```python
from build123d import *

# Parameters (mm, degrees)
SKETCH1_W           = 7.5
SKETCH1_H           = 7.5
BOSS_EXTRUDE1_DEPTH = 7.5
SKETCH2_W           = 5.5
SKETCH2_H           = 6.5
CUT_EXTRUDE1_DEPTH  = 6.5
CUT_EXTRUDE2_REACH  = 13.25
SKETCH4_R           = 1.3
CUT_EXTRUDE3_DEPTH  = 1
SKETCH5_R           = 1.5
CUT_EXTRUDE4_DEPTH  = 0.2
FILLET1_R           = 1


with BuildPart() as part:
    # Sketch1 → Boss-Extrude1 (new body)
    with BuildSketch(Plane(origin=(0, 0, 0), x_dir=(1, 0, 0), z_dir=(0, 1, 0))):
        Rectangle(SKETCH1_W, SKETCH1_H)
    extrude(amount=BOSS_EXTRUDE1_DEPTH)

    # Sketch2 → Cut-Extrude1 (cut)
    with BuildSketch(Plane(origin=(0, 7.5, 0), x_dir=(1, 0, 0), z_dir=(0, 1, 0))):
        with Locations((0, -0.5)):
            Rectangle(SKETCH2_W, SKETCH2_H)
    extrude(amount=-CUT_EXTRUDE1_DEPTH, mode=Mode.SUBTRACT)

    # Cut-Extrude2: up to this face of the body (flat: up to its plane)
    cut_extrude2_end = Plane(part.part.faces().sort_by_distance((-3.75, 3.75, 0))[0])
    # Sketch3 → Cut-Extrude2 (cut, up to the picked face)
    with BuildSketch(Plane(origin=(3.75, 0, 0), x_dir=(0, 0, -1), z_dir=(1, 0, 0)), mode=Mode.PRIVATE) as cut_extrude2_sk1:
        Polygon((-3.75, 7.5), (2.75, 7.5), (-3.75, 1), align=None)
    cut_extrude2_tool1 = split(extrude(cut_extrude2_sk1.sketch, amount=-CUT_EXTRUDE2_REACH, mode=Mode.PRIVATE), bisect_by=cut_extrude2_end, keep=Keep.BOTH, mode=Mode.PRIVATE)
    add(cut_extrude2_tool1.solids().sort_by(Axis((3.75, 5.333333, 1.583333), (-1, 0, 0)))[0], mode=Mode.SUBTRACT)

    # Sketch4 → Cut-Extrude3 (cut)
    with BuildSketch(Plane.XZ):
        with Locations(Location((0, 0, 0), (0, 0, 270))):
            Circle(SKETCH4_R)
    extrude(amount=-CUT_EXTRUDE3_DEPTH, mode=Mode.SUBTRACT)

    # Sketch5 → Cut-Extrude4 (cut)
    with BuildSketch(Plane(origin=(0, 1, 0), x_dir=(1, 0, 0), z_dir=(0, 1, 0))):
        with Locations(Location((0, 0, 0), (0, 0, 270))):
            Circle(SKETCH5_R)
    extrude(amount=-CUT_EXTRUDE4_DEPTH, mode=Mode.SUBTRACT)

    # Fillet1
    fillet1_edges = [part.edges().sort_by_distance(p)[0] for p in [
        (0, 7.5, -3.75),
    ]]
    fillet(fillet1_edges, radius=FILLET1_R - 0.0001)  # a hair under: the kernel refuses the full size


solid = part.part
```
CAD build for the part. Positions are in the model's coordinates, mm. A direction names the side the tool comes from. Coordinates: 2 decimals unless noted, no trailing zeros. Order: outer loops, then holes, each group sorted by start corner. A loop starts at its lowest first (then second) coordinate and runs counter-clockwise, first axis right, second up. Notation, with made-up numbers: (2, 30.25) -> (45, 30.25) arc R20 ccw to (45, 56.25) -> close; hole circle Ø7 at (43, -38). An arc over 180 degrees is marked (long way). Use one line per item in the form item = value. Start each with the question number.
1) Pull direction Z, two halves, no side cores. Call faces 3 (the flat face through (-2.75, 3, -1)), 4 (the cylindrical face through (0.39, 0.39, -1.24)), 5 (the flat face through (-3.24, 4.3, 0.45)): +Z half, -Z half, draft (parallel to the pull), parting line (faces both ways), or undercut.
2) Drill centre lines: L1, parallel to X at y = 3, z = -1; L2, parallel to Z at x = 1.75, y = 1.5; L3, parallel to Y at x = 0.5, z = -1.5. Where is each one in solid material? Low to high. Write a range as [from, to].
3) Band-saw the part on D-D on z = 3.25. Give the cut face in (x, y).
4) Band-saw the part on B-B on z = 0. Give the cut face in (x, y).
5) Band-saw the part on C-C on y = 3.5. Give the cut face in (x, z), then the cut area to 3 significant figures.
6) Drop flat-ended pins along their axis: pin 1 (2.5 mm diameter, centred on x = 0, z = 0, fed in from -Y); pin 2 (3.5 mm diameter, centred on x = 0, z = 0.5, fed in from +Y). Give the stop position or say it passes through.
7) Tool access for faces 1 (the flat face through (3.26, 4.3, 0.45)), 2 (the flat face through (0, 4, -2.75)): list every direction of +Z, -Z, +X, -X, +Y, -Y with a clear straight run to the whole face (end or side of a thin tool).
Entries:
q1.face_3 = draft
q1.face_4 = undercut
q1.face_5 = +Z half
q2.L1 = [-3.75, -2.75], [2.75, 3.75]
q2.L2 = [-3.75, -2.75]
q2.L3 = [0, 1]
q3.outline = (-3.75, 0) -> (3.75, 0) -> (3.75, 1.5) -> (2.75, 1.5) -> (2.75, 1) -> (-2.75, 1) -> (-2.75, 1.5) -> (-3.75, 1.5) -> close
q4.outline = (-3.75, 0) -> (-1.3, 0) -> (-1.3, 0.8) -> (-1.5, 0.8) -> (-1.5, 1) -> (-2.75, 1) -> (-2.75, 4.75) -> (-3.75, 4.75) -> close; (1.3, 0) -> (3.75, 0) -> (3.75, 4.75) -> (2.75, 4.75) -> (2.75, 1) -> (1.5, 1) -> (1.5, 0.8) -> (1.3, 0.8) -> close
q5.outline = (-3.75, -3.75) -> (3.75, -3.75) -> (3.75, 1.25) -> (2.75, 1.25) -> (2.75, -2.75) -> (-2.75, -2.75) -> (-2.75, 1.25) -> (-3.75, 1.25) -> close
q5.area = 15.5 mm2
q6.pin_1 = through
q6.pin_2 = 1
q7.face_1 = +Z, +X, -X, +Y
q7.face_2 = +Z, +Y
